from build123d import *

# Parameters (mm, degrees)
SKETCH_1_W           = 100
SKETCH_1_H           = 80
SKETCH_1_R           = 2.6
EXTRUDE_1_DEPTH      = 9.5
CUT_EXTRUDE_1_DEPTH  = 5.2
EXTRUDE_2_DEPTH      = 25
FILLET_1_R           = 7
SKETCH_7_R           = 20
CUT_EXTRUDE_2_DEPTH  = 99.172361182
EXTRUDE_3_DEPTH      = 2
EXTRUDE_3_DEPTH_BACK = 2


with BuildPart() as part:
    # 草图1 → 凸台-拉伸1 (new body)
    with BuildSketch(Plane(origin=(0, 0, 0), x_dir=(1, 0, 0), z_dir=(0, 1, 0))):
        Rectangle(SKETCH_1_W, SKETCH_1_H)
        with Locations(Location((-45, 30, 0), (0, 0, 270))):
            Circle(SKETCH_1_R, mode=Mode.SUBTRACT)
        with Locations(Location((-5, 30, 0), (0, 0, 270))):
            Circle(SKETCH_1_R, mode=Mode.SUBTRACT)
        with Locations(Location((-5, -30, 0), (0, 0, 270))):
            Circle(SKETCH_1_R, mode=Mode.SUBTRACT)
        with Locations(Location((-45, -30, 0), (0, 0, 270))):
            Circle(SKETCH_1_R, mode=Mode.SUBTRACT)
        with Locations(Location((45, -30, 0), (0, 0, 90))):
            Circle(SKETCH_1_R, mode=Mode.SUBTRACT)
        with Locations(Location((5, -30, 0), (0, 0, 90))):
            Circle(SKETCH_1_R, mode=Mode.SUBTRACT)
        with Locations(Location((5, 30, 0), (0, 0, 90))):
            Circle(SKETCH_1_R, mode=Mode.SUBTRACT)
        with Locations(Location((45, 30, 0), (0, 0, 90))):
            Circle(SKETCH_1_R, mode=Mode.SUBTRACT)
    extrude(amount=EXTRUDE_1_DEPTH)

    # 草图4 → 切除-拉伸1 (cut)
    with BuildSketch(Plane(origin=(0, 9.5, 0), x_dir=(1, 0, 0), z_dir=(0, 1, 0))):
        with BuildLine():
            Line((-5, 34.6), (5, 34.6))
            ThreePointArc((5, 34.6), (9.6, 30), (5, 25.4))
            Line((5, 25.4), (-5, 25.4))
            ThreePointArc((-5, 25.4), (-9.6, 30), (-5, 34.6))
        make_face()
        with BuildLine():
            Line((-5, -25.4), (5, -25.4))
            ThreePointArc((5, -25.4), (9.6, -30), (5, -34.6))
            Line((5, -34.6), (-5, -34.6))
            ThreePointArc((-5, -34.6), (-9.6, -30), (-5, -25.4))
        make_face()
    extrude(amount=-CUT_EXTRUDE_1_DEPTH, mode=Mode.SUBTRACT)

    # 草图5 → 凸台-拉伸2 (add)
    with BuildSketch(Plane(origin=(0, 9.5, 0), x_dir=(1, 0, 0), z_dir=(0, 1, 0))):
        Polygon((-9.6, 27.25), (-9.6, 29.999521433), (-32.75, 29.999521433), (-32.75, -29.999521433), (-9.6, -29.999521433), (-9.6, -27.25), (-30, -27.25), (-30, 27.25), align=None)
        Polygon((32.75, 29.999521433), (9.6, 29.999521433), (9.6, 27.25), (30, 27.25), (30, -27.25), (9.6, -27.25), (9.6, -29.999521433), (32.75, -29.999521433), align=None)
    extrude(amount=EXTRUDE_2_DEPTH)

    # 圆角1
    # the kernel refuses this fillet: 7 mm, written as the material it adds along each edge
    with BuildSketch(Plane(origin=(32.75, 9.5, 29.999521433), x_dir=(1, 0, 0), z_dir=(0, 0, -1)), Plane(origin=(-32.75, 9.5, -29.999521433), x_dir=(-1, 0, 0), z_dir=(0, 0, 1))) as fillet_1_piece_1:
        with BuildLine():
            CenterArc((FILLET_1_R, -FILLET_1_R), FILLET_1_R, 90, 90)
            Line((0, -FILLET_1_R), (-FILLET_1_R * 0.02, -FILLET_1_R))
            Line((-FILLET_1_R * 0.02, -FILLET_1_R), (-FILLET_1_R * 0.02, FILLET_1_R * 0.02))
            Line((-FILLET_1_R * 0.02, FILLET_1_R * 0.02), (FILLET_1_R, FILLET_1_R * 0.02))
            Line((FILLET_1_R, FILLET_1_R * 0.02), (FILLET_1_R, 0))
        make_face()
    extrude(amount=59.999042867)
    with BuildSketch(Plane(origin=(32.75, 9.5, -29.999521433), x_dir=(0, 0, -1), z_dir=(-1, 0, 0)), Plane(origin=(9.6, 9.5, 29.999521433), x_dir=(0, 0, 1), z_dir=(1, 0, 0)), Plane(origin=(-9.6, 9.5, -29.999521433), x_dir=(0, 0, -1), z_dir=(-1, 0, 0)), Plane(origin=(-32.75, 9.5, 29.999521433), x_dir=(0, 0, 1), z_dir=(1, 0, 0))) as fillet_1_piece_2:
        with BuildLine():
            CenterArc((FILLET_1_R, -FILLET_1_R), FILLET_1_R, 90, 90)
            Line((0, -FILLET_1_R), (-FILLET_1_R * 0.02, -FILLET_1_R))
            Line((-FILLET_1_R * 0.02, -FILLET_1_R), (-FILLET_1_R * 0.02, FILLET_1_R * 0.02))
            Line((-FILLET_1_R * 0.02, FILLET_1_R * 0.02), (FILLET_1_R, FILLET_1_R * 0.02))
            Line((FILLET_1_R, FILLET_1_R * 0.02), (FILLET_1_R, 0))
        make_face()
    extrude(amount=23.15)
    with BuildSketch(Plane(origin=(9.6, 9.5, 29.999521433), x_dir=(0, 0, 1), z_dir=(1, 0, 0))) as fillet_1_piece_3a_section:
        with BuildLine():
            CenterArc((FILLET_1_R, -FILLET_1_R), FILLET_1_R, 90, 90)
            Line((0, -FILLET_1_R), (-FILLET_1_R * 0.02, -FILLET_1_R))
            Line((-FILLET_1_R * 0.02, -FILLET_1_R), (-FILLET_1_R * 0.02, FILLET_1_R * 0.02))
            Line((-FILLET_1_R * 0.02, FILLET_1_R * 0.02), (FILLET_1_R, FILLET_1_R * 0.02))
            Line((FILLET_1_R, FILLET_1_R * 0.02), (FILLET_1_R, 0))
        make_face()
    fillet_1_piece_3a = extrude(amount=40.65, mode=Mode.PRIVATE)
    fillet_1_piece_3a = split(fillet_1_piece_3a, bisect_by=Plane(origin=(32.75, 11.0847658, 31.584287233), z_dir=(1, 0, 0)), keep=Keep.TOP, mode=Mode.PRIVATE)
    with BuildSketch(Plane(origin=(32.75, 9.5, 47.499521433), x_dir=(1, 0, 0), z_dir=(0, 0, -1))) as fillet_1_piece_3b_section:
        with BuildLine():
            CenterArc((FILLET_1_R, -FILLET_1_R), FILLET_1_R, 90, 90)
            Line((0, -FILLET_1_R), (-FILLET_1_R * 0.02, -FILLET_1_R))
            Line((-FILLET_1_R * 0.02, -FILLET_1_R), (-FILLET_1_R * 0.02, FILLET_1_R * 0.02))
            Line((-FILLET_1_R * 0.02, FILLET_1_R * 0.02), (FILLET_1_R, FILLET_1_R * 0.02))
            Line((FILLET_1_R, FILLET_1_R * 0.02), (FILLET_1_R, 0))
        make_face()
    fillet_1_piece_3b = extrude(amount=77.499042867, mode=Mode.PRIVATE)
    fillet_1_piece_3b = split(fillet_1_piece_3b, bisect_by=Plane(origin=(34.3347658, 11.0847658, 29.999521433), z_dir=(0, 0, 1)), keep=Keep.TOP, mode=Mode.PRIVATE)
    fillet_1_piece_3 = fillet_1_piece_3a & fillet_1_piece_3b
    add(fillet_1_piece_3)
    with BuildSketch(Plane(origin=(32.75, 9.5, 29.999521433), x_dir=(1, 0, 0), z_dir=(0, 0, -1))) as fillet_1_piece_4a_section:
        with BuildLine():
            CenterArc((FILLET_1_R, -FILLET_1_R), FILLET_1_R, 90, 90)
            Line((0, -FILLET_1_R), (-FILLET_1_R * 0.02, -FILLET_1_R))
            Line((-FILLET_1_R * 0.02, -FILLET_1_R), (-FILLET_1_R * 0.02, FILLET_1_R * 0.02))
            Line((-FILLET_1_R * 0.02, FILLET_1_R * 0.02), (FILLET_1_R, FILLET_1_R * 0.02))
            Line((FILLET_1_R, FILLET_1_R * 0.02), (FILLET_1_R, 0))
        make_face()
    fillet_1_piece_4a = extrude(amount=77.499042867, mode=Mode.PRIVATE)
    fillet_1_piece_4a = split(fillet_1_piece_4a, bisect_by=Plane(origin=(34.3347658, 11.0847658, -29.999521433), z_dir=(0, 0, -1)), keep=Keep.TOP, mode=Mode.PRIVATE)
    with BuildSketch(Plane(origin=(50.25, 9.5, -29.999521433), x_dir=(0, 0, -1), z_dir=(-1, 0, 0))) as fillet_1_piece_4b_section:
        with BuildLine():
            CenterArc((FILLET_1_R, -FILLET_1_R), FILLET_1_R, 90, 90)
            Line((0, -FILLET_1_R), (-FILLET_1_R * 0.02, -FILLET_1_R))
            Line((-FILLET_1_R * 0.02, -FILLET_1_R), (-FILLET_1_R * 0.02, FILLET_1_R * 0.02))
            Line((-FILLET_1_R * 0.02, FILLET_1_R * 0.02), (FILLET_1_R, FILLET_1_R * 0.02))
            Line((FILLET_1_R, FILLET_1_R * 0.02), (FILLET_1_R, 0))
        make_face()
    fillet_1_piece_4b = extrude(amount=40.65, mode=Mode.PRIVATE)
    fillet_1_piece_4b = split(fillet_1_piece_4b, bisect_by=Plane(origin=(32.75, 11.0847658, -31.584287233), z_dir=(1, 0, 0)), keep=Keep.TOP, mode=Mode.PRIVATE)
    fillet_1_piece_4 = fillet_1_piece_4a & fillet_1_piece_4b
    add(fillet_1_piece_4)
    with BuildSketch(Plane(origin=(-9.6, 9.5, -29.999521433), x_dir=(0, 0, -1), z_dir=(-1, 0, 0))) as fillet_1_piece_5a_section:
        with BuildLine():
            CenterArc((FILLET_1_R, -FILLET_1_R), FILLET_1_R, 90, 90)
            Line((0, -FILLET_1_R), (-FILLET_1_R * 0.02, -FILLET_1_R))
            Line((-FILLET_1_R * 0.02, -FILLET_1_R), (-FILLET_1_R * 0.02, FILLET_1_R * 0.02))
            Line((-FILLET_1_R * 0.02, FILLET_1_R * 0.02), (FILLET_1_R, FILLET_1_R * 0.02))
            Line((FILLET_1_R, FILLET_1_R * 0.02), (FILLET_1_R, 0))
        make_face()
    fillet_1_piece_5a = extrude(amount=40.65, mode=Mode.PRIVATE)
    fillet_1_piece_5a = split(fillet_1_piece_5a, bisect_by=Plane(origin=(-32.75, 11.0847658, -31.584287233), z_dir=(-1, 0, 0)), keep=Keep.TOP, mode=Mode.PRIVATE)
    with BuildSketch(Plane(origin=(-32.75, 9.5, -47.499521433), x_dir=(-1, 0, 0), z_dir=(0, 0, 1))) as fillet_1_piece_5b_section:
        with BuildLine():
            CenterArc((FILLET_1_R, -FILLET_1_R), FILLET_1_R, 90, 90)
            Line((0, -FILLET_1_R), (-FILLET_1_R * 0.02, -FILLET_1_R))
            Line((-FILLET_1_R * 0.02, -FILLET_1_R), (-FILLET_1_R * 0.02, FILLET_1_R * 0.02))
            Line((-FILLET_1_R * 0.02, FILLET_1_R * 0.02), (FILLET_1_R, FILLET_1_R * 0.02))
            Line((FILLET_1_R, FILLET_1_R * 0.02), (FILLET_1_R, 0))
        make_face()
    fillet_1_piece_5b = extrude(amount=77.499042867, mode=Mode.PRIVATE)
    fillet_1_piece_5b = split(fillet_1_piece_5b, bisect_by=Plane(origin=(-34.3347658, 11.0847658, -29.999521433), z_dir=(0, 0, -1)), keep=Keep.TOP, mode=Mode.PRIVATE)
    fillet_1_piece_5 = fillet_1_piece_5a & fillet_1_piece_5b
    add(fillet_1_piece_5)
    with BuildSketch(Plane(origin=(-32.75, 9.5, -29.999521433), x_dir=(-1, 0, 0), z_dir=(0, 0, 1))) as fillet_1_piece_6a_section:
        with BuildLine():
            CenterArc((FILLET_1_R, -FILLET_1_R), FILLET_1_R, 90, 90)
            Line((0, -FILLET_1_R), (-FILLET_1_R * 0.02, -FILLET_1_R))
            Line((-FILLET_1_R * 0.02, -FILLET_1_R), (-FILLET_1_R * 0.02, FILLET_1_R * 0.02))
            Line((-FILLET_1_R * 0.02, FILLET_1_R * 0.02), (FILLET_1_R, FILLET_1_R * 0.02))
            Line((FILLET_1_R, FILLET_1_R * 0.02), (FILLET_1_R, 0))
        make_face()
    fillet_1_piece_6a = extrude(amount=77.499042867, mode=Mode.PRIVATE)
    fillet_1_piece_6a = split(fillet_1_piece_6a, bisect_by=Plane(origin=(-34.3347658, 11.0847658, 29.999521433), z_dir=(0, 0, 1)), keep=Keep.TOP, mode=Mode.PRIVATE)
    with BuildSketch(Plane(origin=(-50.25, 9.5, 29.999521433), x_dir=(0, 0, 1), z_dir=(1, 0, 0))) as fillet_1_piece_6b_section:
        with BuildLine():
            CenterArc((FILLET_1_R, -FILLET_1_R), FILLET_1_R, 90, 90)
            Line((0, -FILLET_1_R), (-FILLET_1_R * 0.02, -FILLET_1_R))
            Line((-FILLET_1_R * 0.02, -FILLET_1_R), (-FILLET_1_R * 0.02, FILLET_1_R * 0.02))
            Line((-FILLET_1_R * 0.02, FILLET_1_R * 0.02), (FILLET_1_R, FILLET_1_R * 0.02))
            Line((FILLET_1_R, FILLET_1_R * 0.02), (FILLET_1_R, 0))
        make_face()
    fillet_1_piece_6b = extrude(amount=40.65, mode=Mode.PRIVATE)
    fillet_1_piece_6b = split(fillet_1_piece_6b, bisect_by=Plane(origin=(-32.75, 11.0847658, 31.584287233), z_dir=(-1, 0, 0)), keep=Keep.TOP, mode=Mode.PRIVATE)
    fillet_1_piece_6 = fillet_1_piece_6a & fillet_1_piece_6b
    add(fillet_1_piece_6)

    # 草图7 → 切除-拉伸2 (cut, through all)
    with BuildSketch(Plane.ZY.offset(32.75)):
        with Locations((0, 46.25)):
            Circle(SKETCH_7_R)
    extrude(amount=-CUT_EXTRUDE_2_DEPTH, mode=Mode.SUBTRACT)

    # 草图6 → 凸台-拉伸3 (add, two sides: drawn at the far end of the back side and taken through both)
    with BuildSketch(Plane.XY.offset(-EXTRUDE_3_DEPTH_BACK)):
        Polygon((-32.75, 26.25), (-50, 9.5), (-32.75, 9.5), align=None)
        Polygon((32.75, 9.5), (32.75, 26.25), (50, 9.5), align=None)
    extrude(amount=EXTRUDE_3_DEPTH + EXTRUDE_3_DEPTH_BACK)


solid = part.part
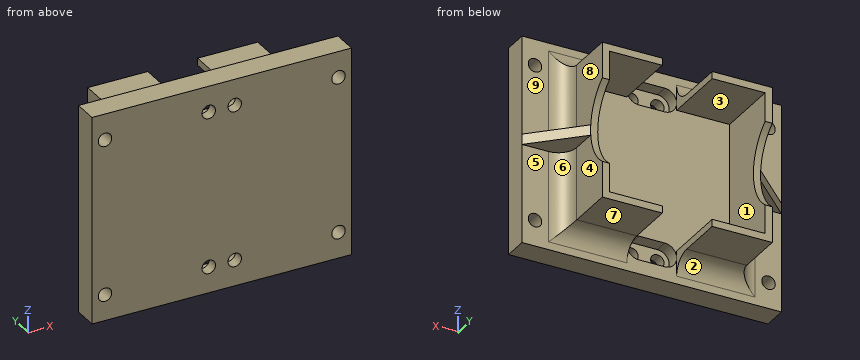
For this review, take the finished solid that the model builds, in its own axes (mm). Face numbers are marked on the shaded views. A direction names the side the tool comes from. Round coordinates to 2 decimals unless told otherwise and drop trailing zeros. Order: outer loops, then holes, each group sorted by start corner. A loop starts at its lowest first (then second) coordinate and runs counter-clockwise, first axis right, second up. Notation, with made-up numbers: (29.25, 30) -> (74.25, 30) arc R30 cw to (74.25, 66) -> close; hole circle Ø2 at (76.25, 45.5). An arc over 180 degrees is marked (long way). Write item = value, one per line. Start each with the question number.
1) Take a section at B-B on x = 15.5. State the section outline as (y, z) points, plus the area to 3 significant figures.
2) Take a section at D-D on x = -45. State the section outline as (y, z) points.
3) The part is to be moulded in two halves that separate along X. For the marked faces 1, 2, 3 and 4, say which applies: +X half, -X half, draft (parallel to the pull), parting line (faces both ways), or undercut.
4) To check wall thickness, follow line 1 (Z direction, x = -5, y = 3); line 2 (X direction, y = 1.5, z = 30); line 3 (X direction, y = 5, z = -30). State the ranges of each line that lie inside material, in increasing order. Write a range as from..to.
5) Take a section at A-A on y = 12. State the section outline as (x, z) points.
6) Tool access review of the marked faces 5, 6, 7, 8 and 9: name each direction out of +Z, -Z, +X, -X, +Y, -Y from which nothing blocks a thin tool from reaching the whole face with its end or side.
7) Take a section at C-C on z = 5.5. State the section outline as (x, y) points, plus the area to 3 significant figures.
8) Insertion check: pin 1 (6 mm diameter, centred on x = 5, z = -30, fed in from +Y); pin 2 (10.5 mm diameter, centred on y = 20, z = -34, fed in from +X); pin 3 (10 mm diameter, centred on x = 21, y = 27, fed in from -Z); pin 4 (5 mm diameter, centred on y = 24.5, z = -34.5, fed in from -X). Each pin has a flat end and moves straight along its axis. Give the tip position at first contact, or say it passes through.
Verdict:
q1.outline = (0, -40) -> (9.5, -40) -> (9.5, -37) arc R7 cw to (16.5, -30) -> (34.5, -30) -> (34.5, -27.25) -> (9.5, -27.25) -> (9.5, 27.25) -> (34.5, 27.25) -> (34.5, 30) -> (16.5, 30) arc R7 cw to (9.5, 37) -> (9.5, 40) -> (0, 40) -> close
q1.area = 919 mm2
q2.outline = (0, -40) -> (9.5, -40) -> (9.5, -32.6) -> (0, -32.6) -> close; (0, -27.4) -> (9.5, -27.4) -> (9.5, -2) -> (14.36, -2) -> (14.36, 2) -> (9.5, 2) -> (9.5, 27.4) -> (0, 27.4) -> close; (0, 32.6) -> (9.5, 32.6) -> (9.5, 40) -> (0, 40) -> close
q3.face_1 = undercut
q3.face_2 = draft
q3.face_3 = undercut
q3.face_4 = +X half
q4.line_1 = -40..-32.6, -27.4..27.4, 32.6..40
q4.line_2 = -50..-47.6, -42.4..-7.6, -2.4..2.4, 7.6..42.4, 47.6..50
q4.line_3 = -50..-47.6, -42.4..-9.6, 9.6..42.4, 47.6..50
q5.outline = (-47.43, -2) -> (-34.39, -2) -> (-34.39, -31.64) -> (-9.6, -31.64) -> (-9.6, -27.25) -> (-30, -27.25) -> (-30, 27.25) -> (-9.6, 27.25) -> (-9.6, 31.64) -> (-34.39, 31.64) -> (-34.39, 2) -> (-47.43, 2) -> close; (9.6, -31.64) -> (34.39, -31.64) -> (34.39, -2) -> (47.43, -2) -> (47.43, 2) -> (34.39, 2) -> (34.39, 31.64) -> (9.6, 31.64) -> (9.6, 27.25) -> (30, 27.25) -> (30, -27.25) -> (9.6, -27.25) -> close
q6.face_5 = -Z, +Y
q6.face_6 = -Z, +X, +Y
q6.face_7 = -Z, +X, -X, +Y
q6.face_8 = +Z, +X, +Y
q6.face_9 = +Z, +Y
q7.outline = (-50, 0) -> (50, 0) -> (50, 9.5) -> (39.75, 9.5) arc R7 cw to (32.75, 16.5) -> (32.75, 27.02) -> (30, 27.02) -> (30, 9.5) -> (-30, 9.5) -> (-30, 27.02) -> (-32.75, 27.02) -> (-32.75, 16.5) arc R7 cw to (-39.75, 9.5) -> (-50, 9.5) -> close
q7.area = 1,070 mm2
q8.pin_1 = 4.3
q8.pin_2 = 32.75
q8.pin_3 = -30
q8.pin_4 = through
